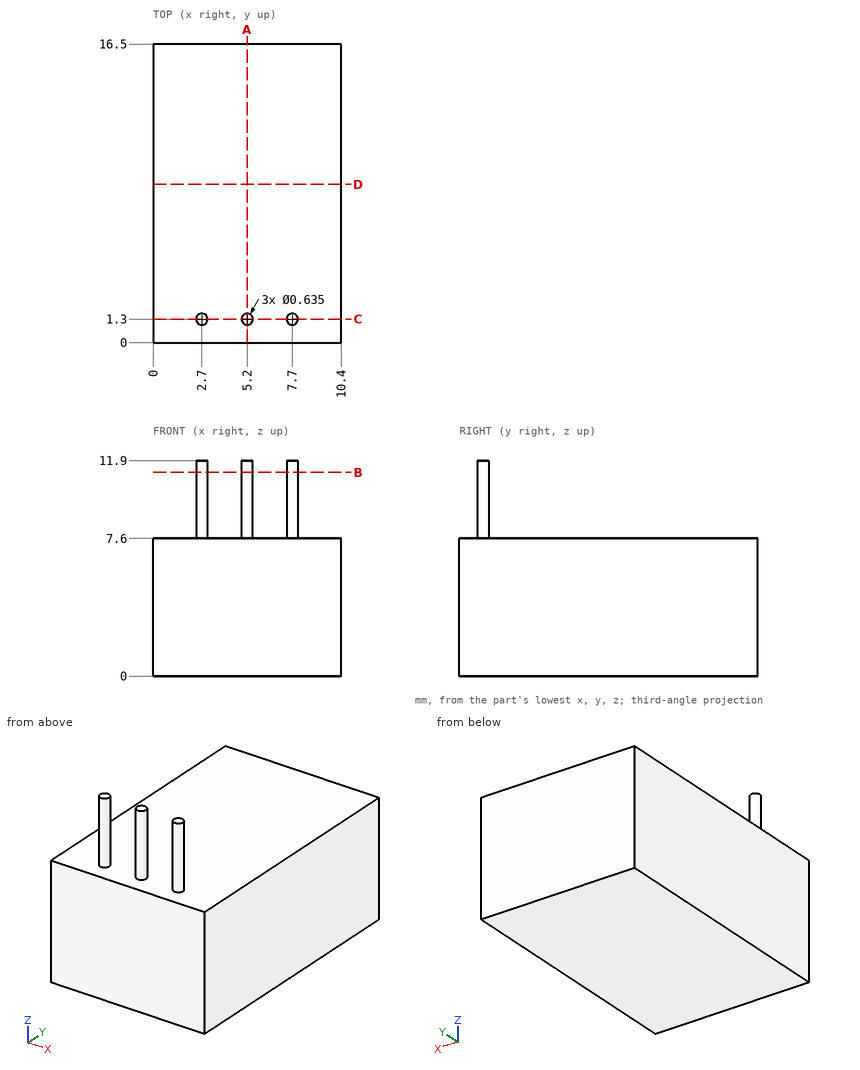
Input: dimensioned drawing with shaded views. Units: mm. Origin: part minimum x, y, z. Coordinates: 2 decimals unless noted, no trailing zeros. Order: outer loops, then holes, each group sorted by start corner. A loop starts at its lowest first (then second) coordinate and runs counter-clockwise, first axis right, second up. Notation, with made-up numbers: M 59,49.25 L 80,49.25 A15 cw 80,53.25 Z; hole C 58,13 d7. An arc over 180 degrees is marked long. Write each question's results on one line, items separated by ' | '. Start each with the question number.
Item 1: Cut plane D-D (y = 8.75). Return loops of the section in (x, z), and give its area (3 significant figures).
Item 2: Line query: probe 1 along Z at (x, y) = (2.5, 15.5). Output: solid intervals per line, ascending.
Item 3: Cut plane B-B (z = 11.25). Return loops of the section in (x, y) (1 decimal).
Item 4: Cut plane C-C (y = 1.3). Return loops of the section in (x, z).
Item 5: Cut plane A-A (x = 5.2). Return loops of the section in (y, z).
Checked values:
1) outline: M 0,0 L 10.4,0 L 10.4,7.6 L 0,7.6 Z | area: 79.0 mm2
2) probe 1: z = 0 to 7.6
3) outline: C 2.7,1.3 d0.6; C 5.2,1.3 d0.6; C 7.7,1.3 d0.6
4) outline: M 0,0 L 10.4,0 L 10.4,7.6 L 8.02,7.6 L 8.02,11.9 L 7.38,11.9 L 7.38,7.6 L 5.52,7.6 L 5.52,11.9 L 4.88,11.9 L 4.88,7.6 L 3.02,7.6 L 3.02,11.9 L 2.38,11.9 L 2.38,7.6 L 0,7.6 Z
5) outline: M 0,0 L 16.5,0 L 16.5,7.6 L 1.62,7.6 L 1.62,11.9 L 0.98,11.9 L 0.98,7.6 L 0,7.6 Z
